from build123d import *

# Parameters (mm, degrees)
F0_W      = 44.45
F0_H      = 10.16
F1_DEPTH  = 25.4
F3_DEPTH  = 10.16
F4_W      = 12.7
F4_H      = 25.4
F5_DEPTH  = 19.05
F6_DEPTH  = 6.35
F9_DEPTH  = 25.4
F10_DEPTH = 25.4
F11_DEPTH = 50.8
F12_W     = 12.7
F12_H     = 12.7
F13_DEPTH = 25.4
F14_R     = 6.35
F15_DEPTH = 25.4
F16_R     = 6.35
F17_DEPTH = 25.4


with BuildPart() as f1:
    # F0 (on Front) → F1 (new body)
    with BuildSketch(Plane.XZ):
        with Locations((-22.225, 5.08)):
            Rectangle(F0_W, F0_H)
    extrude(amount=F1_DEPTH)

    # F2 (on face) → F3 (join)
    with BuildSketch(Plane.XY.offset(10.16)):
        with BuildLine():
            Line((0, 0), (0, -25.4))
            ThreePointArc((0, -25.4), (12.7, -12.7), (0, 0))
        make_face()
    extrude(amount=-F3_DEPTH)

    # F4 (on face) → F5 (join)
    with BuildSketch(Plane.XY.offset(10.16)):
        with Locations((-38.1, -12.7)):
            Rectangle(F4_W, F4_H)
    extrude(amount=F5_DEPTH)

    # F6 (add): a face of the model
    f6_faces = [f1.faces().sort_by_distance(p)[0] for p in [
        (-38.1, -12.7, 29.21),
    ]]
    extrude(f6_faces, amount=F6_DEPTH)

    # F7 (on face) → F9 (cut)
    with BuildSketch(Plane.YZ.offset(-31.75)):
        with BuildLine():
            ThreePointArc((-25.4, 29.21), (-23.1840796039, 33.3440796039), (-19.05, 35.56))
            Line((-19.05, 35.56), (-25.4, 35.56))
            Line((-25.4, 35.56), (-25.4, 29.21))
        make_face()
    extrude(amount=-F9_DEPTH, mode=Mode.SUBTRACT)

    # F8 (on face) → F10 (join)
    with BuildSketch(Plane.YZ.offset(-31.75)):
        with BuildLine():
            ThreePointArc((-6.35, 35.56), (-2.4561746111, 33.1038253889), (0, 29.21))
            Line((0, 29.21), (0, 35.56))
            Line((0, 35.56), (-6.35, 35.56))
        make_face()
    extrude(amount=F10_DEPTH)

    # F11 (cut): a face of the model
    f11_faces = [f1.faces().sort_by_distance(p)[0] for p in [
        (-6.35, -1.7790367602, 33.7809632398),
    ]]
    extrude(f11_faces, amount=-F11_DEPTH, mode=Mode.SUBTRACT)

    # F12 (on face) → F13 (cut)
    with BuildSketch(Plane.YZ.offset(-31.75)):
        with Locations((-12.7, 29.21)):
            Rectangle(F12_W, F12_H)
        with BuildLine():
            Line((-6.35, 22.86), (-19.05, 22.86))
            ThreePointArc((-19.05, 22.86), (-12.7, 16.51), (-6.35, 22.86))
        make_face()
    extrude(amount=-F13_DEPTH, mode=Mode.SUBTRACT)

    # F14 (on face) → F15 (cut)
    with BuildSketch(Plane.XY.offset(10.16)):
        with Locations((-19.05, -12.7)):
            Circle(F14_R)
    extrude(amount=-F15_DEPTH, mode=Mode.SUBTRACT)

    # F16 (on face) → F17 (cut)
    with BuildSketch(Plane.XY.offset(10.16)):
        with Locations((0, -12.7)):
            Circle(F16_R)
    extrude(amount=-F17_DEPTH, mode=Mode.SUBTRACT)


solid = f1.part
Design review of the part built by this model. Coordinates are the model's own, in mm. A direction names the side the tool comes from. Round coordinates to 2 decimals unless told otherwise and drop trailing zeros. Write each loop counter-clockwise with the first axis right and the second up, starting at its lowest first coordinate (ties: lowest second). Pieces come first, ordered by that corner, then holes. Notation, with made-up numbers: (9.25, 51.25) -> (56.25, 51.25) arc R23 cw to (56.25, 85.25) -> close; hole circle Ø3 at (-10, 0). An arc over 180 degrees is marked (long way). One line per question, with ' | ' between items.
(1) Machinability: for faces 5 (the flat face through (-38, -6.35, 29)), 6 (the cylindrical face through (12.697, -12.979, 5.151)), 7 (the flat face through (-31.75, -16, 17)), which of the approach directions +Z, -Z, +X, -X, +Y, -Y give a long, thin tool a straight path to every point of the face, cutting with its end or side? Answer none if there is none.
Result sheet:
face 5: +Z, +X, -X | face 6: +Z, -Z, +X | face 7: +Z, +X, +Y, -Y
(2) Take a section at A-A, the plane x = -19.05. State the section outline as (y, z) points.
Result sheet:
outline: (-25.4, 0) -> (-19.05, 0) -> (-19.05, 10.16) -> (-25.4, 10.16) -> close; (-6.35, 0) -> (0, 0) -> (0, 10.16) -> (-6.35, 10.16) -> close
(3) Wall thickness on line 1 (Y direction, x = -19, z = 5); line 2 (X direction, y = -8, z = 10): over which ranges is each line inside the solid? List them lowest first. Write a range as [from, to].
Result sheet:
line 1: [-25.4, -19.05], [-6.35, 0] | line 2: [-44.45, -23.32], [-14.78, -4.27], [4.27, 11.8]
(4) Insertion check: P1, Ø10, axis at y = -18, z = 21.5, coming from the +X side; P2, Ø4, axis at y = -22.5, z = 6, coming from the +X side. Each pin has a flat end and moves straight along its axis. Give the tip position at first contact, or say it passes through.
Result sheet:
P1: x = -31.75 | P2: x = 10.02
(5) Take a section at C-C, the plane z = 17.5. State the section outline as (x, y) points.
Result sheet:
outline: (-44.45, -25.4) -> (-31.75, -25.4) -> (-31.75, -16.1) -> (-44.45, -16.1) -> close; (-44.45, -9.3) -> (-31.75, -9.3) -> (-31.75, 0) -> (-44.45, 0) -> close
(6) Take a section at D-D, the plane z = 9. State the section outline as (x, y) points, and give its area (3 significant figures).
Result sheet:
outline: (-44.45, -25.4) -> (0, -25.4) arc R12.7 ccw to (0, 0) -> (-44.45, 0) -> close; hole circle Ø12.7 at (-19.05, -12.7); hole circle Ø12.7 at (0, -12.7) | area: 1,130 mm2
(7) Take a section at B-B, the plane y = -12.7. State the section outline as (x, z) points.
Result sheet:
outline: (-44.45, 0) -> (-25.4, 0) -> (-25.4, 10.16) -> (-31.75, 10.16) -> (-31.75, 16.51) -> (-44.45, 16.51) -> close; (-12.7, 0) -> (-6.35, 0) -> (-6.35, 10.16) -> (-12.7, 10.16) -> close; (6.35, 0) -> (12.7, 0) -> (12.7, 10.16) -> (6.35, 10.16) -> close
(8) Draft analysis for pull direction Y (two halves, no side actions). For faces 1 (the cylindrical face through (-24.09, -16.56, 5.15)), 2 (the cylindrical face through (-1.38, -18.9, 5.15)), 3 (the flat face through (-27, 0, 8)), 4 (the flat face through (-10, -13, 10.16)), state which applies: released by +Y, released by -Y, zero draft, split by the parting line, or undercut.
Result sheet:
face 1: undercut | face 2: undercut | face 3: released by +Y | face 4: zero draft
